```python
from build123d import *

# Parameters (mm, degrees)
BOSS_EXTRUDE1_DEPTH = 1.5
SKETCH2_W           = 3
SKETCH2_H           = 10
CUT_EXTRUDE1_DEPTH  = 58.801384066
CUT_EXTRUDE3_DEPTH  = 58.801384066
CUT_EXTRUDE4_DEPTH  = 58.801384066
SKETCH6_W           = 18.566482568
SKETCH6_H           = 17.933193013
BOSS_EXTRUDE3_DEPTH = 3


with BuildPart() as part:
    # Sketch1 → Boss-Extrude1 (new, symmetric)
    with BuildSketch(Plane.XY):
        Polygon((-20, -11), (20, -11), (20, -14), (35, -14), (35, -11), (56, -11), (56, 11), (-56, 11), (-56, -11), (-35, -11), (-35, -14), (-20, -14), align=None)
    extrude(amount=BOSS_EXTRUDE1_DEPTH, both=True)

    # Sketch2 → Cut-Extrude1 (cut, through all)
    with BuildSketch(Plane.XY.offset(1.5)):
        with Locations((2.5, 0)):
            Rectangle(SKETCH2_W, SKETCH2_H)
        with Locations((52.5, 0)):
            Rectangle(SKETCH2_W, SKETCH2_H)
    extrude(amount=-CUT_EXTRUDE1_DEPTH, mode=Mode.SUBTRACT)

    # Sketch4 → Cut-Extrude3 (cut, through all)
    with BuildSketch(Plane.XY.offset(1.5)):
        Polygon((25, 11), (25, 4), (23.5, 4), (23.5, 0), (25, 0), (25, -4), (30, -4), (30, 0), (31.5, 0), (31.5, 4), (30, 4), (30, 11), align=None)
        Polygon((-30, 11), (-25, 11), (-25, 4), (-23.5, 4), (-23.5, 0), (-25, 0), (-25, -4), (-30, -4), (-30, 0), (-31.5, 0), (-31.5, 4), (-30, 4), align=None)
    extrude(amount=-CUT_EXTRUDE3_DEPTH, mode=Mode.SUBTRACT)

    # Sketch5 → Cut-Extrude4 (cut, through all)
    with BuildSketch(Plane.XY.offset(1.5)):
        Polygon((-51.5, 11), (-51.5, 4), (-52.75, 4), (-52.75, 1), (-51.5, 1), (-51.5, -3), (-48.5, -3), (-48.5, 1), (-47.25, 1), (-47.25, 4), (-48.5, 4), (-48.5, 11), align=None)
        Polygon((48.5, 11), (51.5, 11), (51.5, 4), (52.75, 4), (52.75, 1), (51.5, 1), (51.5, -3), (48.5, -3), (48.5, 1), (47.25, 1), (47.25, 4), (48.5, 4), align=None)
    extrude(amount=-CUT_EXTRUDE4_DEPTH, mode=Mode.SUBTRACT)

    # Sketch6 → Boss-Extrude3 (add, through all)
    with BuildSketch(Plane.XY.offset(1.5)):
        with Locations((-26.473921785, 2.033403493)):
            Rectangle(SKETCH6_W, SKETCH6_H)
    extrude(amount=-BOSS_EXTRUDE3_DEPTH)


solid = part.part
```
CAD build for the part. Positions are in the model's coordinates, mm. A direction names the side the tool comes from. Round coordinates to 2 decimals unless told otherwise and drop trailing zeros. Write each loop counter-clockwise with the first axis right and the second up, starting at its lowest first coordinate (ties: lowest second). Pieces come first, ordered by that corner, then holes. Notation, with made-up numbers: (-2.75, 7.25) -> (22.25, 7.25) arc R27 ccw to (22.25, 30.25) -> close; hole circle Ø5 at (56.25, 20). An arc over 180 degrees is marked (long way). Answer in a Markdown table with one row per item. Add a question column.
Item 1: Saw through at A-A, the plane y = -12.25. Write the cut outline in (x, z).
Item 2: Drill centre lines: line 1 (X direction, y = 1.25, z = -0.1); line 2 (X direction, y = -2.5, z = 0.1); line 3 (X direction, y = 6, z = -0.5). Where is each one in solid material? Low to high. Write a range as from..to.
Item 3: Mould opens along X. For faces 1 (the face through (39, 11, 0)), 2 (the face through (25, 8, 0)) say: pulls with the +X half, pulls with the -X half, needs draft (parallel to the pull), parting line crosses it, or undercut.
Item 4: Drop flat-ended pins along their axis: pin 1 Ø0.9 at (x, z) = (50, 0) entering from -Y; pin 2 Ø1.5 at (y, z) = (-12.5, -0.5) entering from +X. Give the stop position or say it passes through.
Item 5: Which spindle directions (+Z, -Z, +X, -X, +Y, -Y) get a long thin tool onto all of the face, cutting with end or side? Do faces 3 (the face through (20, -12, 0)), 4 (the face through (48.5, -1, 0)), 5 (the face through (27, -14, 0)), 6 (the face through (-1, -1, -1.5)), 7 (the face through (54, 0, 0)). Say none if no direction does.
Item 6: Saw through at B-B, the plane x = -5. Write the cut outline in (y, z).
Findings below:
| question | item | result |
|---|---|---|
| 1 | outline | (-35, -1.5) -> (-20, -1.5) -> (-20, 1.5) -> (-35, 1.5) -> close; (20, -1.5) -> (35, -1.5) -> (35, 1.5) -> (20, 1.5) -> close |
| 2 | line 1 | x = -56..-52.75, -47.25..1, 4..23.5, 31.5..47.25, 54..56 |
| 2 | line 2 | x = -56..-51.5, -48.5..1, 4..25, 30..48.5, 54..56 |
| 2 | line 3 | x = -56..-51.5, -48.5..25, 30..48.5, 51.5..56 |
| 3 | face 1 | needs draft |
| 3 | face 2 | undercut |
| 4 | pin 1 | stops at y = -11 |
| 4 | pin 2 | stops at x = 35 |
| 5 | face 3 | +Z, -Z, -Y |
| 5 | face 4 | +Z, -Z, +Y |
| 5 | face 5 | +Z, -Z, +X, -X, -Y |
| 5 | face 6 | -Z, +X, -X, +Y, -Y |
| 5 | face 7 | +Z, -Z |
| 6 | outline | (-11, -1.5) -> (11, -1.5) -> (11, 1.5) -> (-11, 1.5) -> close |
